Autodesk Inventor part; units mm, degrees
ref_plane "YZ Plane" through (0, 0, 0) normal (1, 0, 0) x (0, 1, 0)
ref_plane "XZ Plane" through (0, 0, 0) normal (0, 1, 0) x (-1, 0, 0)
ref_plane "XY Plane" through (0, 0, 0) normal (0, 0, 1) x (1, 0, 0)
sketch "スケッチ1" plane through (0, 0, 0) normal (0, 0, 1) x (1, 0, 0)
  line L0 (-22.5, -5) -> (22.5, -5)
  line L1 (22.5, -5) -> (22.5, 5)
  line L2 (22.5, 5) -> (-22.5, 5)
  line L3 (-22.5, 5) -> (-22.5, -5)
  line L4 (-22.5, -5) -> (22.5, 5) construction
  line L5 (22.5, -5) -> (-22.5, 5) construction
  point P0 (0, 0)
  dimension "d0" = 45
  dimension "d1" = 10
extrude "押し出し1" add sketch "スケッチ1" along normal mid plane 55
sketch "スケッチ2" plane through (0, 0, 27.5) normal (0, 0, 1) x (1, 0, 0)
  line L0 (22.5, 5) -> (-22.5, 5)
  line L1 (-22.5, 5) -> (-22.5, -5)
  line L2 (22.5, -5) -> (22.5, 5)
  point P0 (0, 0)
  point P1 (-17.5, 0)
  point P2 (17.5, 0)
  dimension "d4" = 5
  dimension "d5" = 5
  dimension "d6" = 5
  dimension "d7" = 5
hole "穴1" at (-17.5, 0, 27.5) at (17.5, 0, 27.5) direction (0, 0, -1) diameter 2.459 depth 8.8 tip angle 118
sketch "スケッチ3" plane through (0, 0, -27.5) normal (0, 0, -1) x (-1, 0, 0)
  line L0 (-22.5, 5) -> (-22.5, -5)
  line L1 (-22.5, -5) -> (22.5, -5)
  line L2 (22.5, -5) -> (22.5, 5)
  line L3 (22.5, 5) -> (-22.5, 5)
  circle A0 centre (-17.5, 0) radius 1.2295
  circle A1 centre (17.5, 0) radius 1.2295
  point P0 (0, 0)
hole "穴2" at (17.5, 0, -27.5) at (-17.5, 0, -27.5) direction (0, 0, 1) diameter 2.459 depth 8.8 tip angle 118
sketch "スケッチ4" plane through (-22.5, 5, 27.5) normal (0, 1, 0) x (1, 0, 0)
  line L0 (45, 55) -> (45, 0)
  line L1 (45, 0) -> (0, 0)
  point P0 (22.5, 27.5)
  point P1 (33, 27.5)
  dimension "d22" = 12
  dimension "d23" = 27.5
hole "穴3" at (10.5, 5, 0) direction (0, -1, 0) diameter 6.4 end through all
sketch "スケッチ5" plane through (0, 0, 27.5) normal (0, 0, 1) x (1, 0, 0)
  circle A0 centre (17.5, 0) radius 1.2295
  circle A1 centre (-17.5, 0) radius 1.2295
  line L0 (22.5, -5) -> (22.5, 5)
  line L1 (22.5, 5) -> (-22.5, 5)
  line L2 (-22.5, 5) -> (-22.5, -5)
  line L3 (-22.5, -5) -> (22.5, -5)
  line L4 (-17.5, 0) -> (17.5, 0) construction
  line L5 (-17.5, -5) -> (17.5, -5)
  line L6 (17.5, 5) -> (-17.5, 5)
  arc A2 (-17.5, 5) -> (-17.5, -5) centre (-17.5, 0) ccw
  arc A3 (17.5, -5) -> (17.5, 5) centre (17.5, 0) ccw
  point P0 (0, 0)
  point P1 (0, 0)
  point P2 (22.5, 0)
  point P3 (-22.5, 0)
extrude "押し出し2" cut sketch "スケッチ5" against normal through all contours L3 A3 L0 | A3 L1 L0 | L3 L2 A2 | A2 L2 L1
properties part number "camera_connect_part"
For this review, take the finished solid that the model builds, in its own axes (mm). A direction names the side the tool comes from. Coordinates: 2 decimals unless noted, no trailing zeros. Loops run counter-clockwise (first coordinate to the right, second up) from the corner with the lowest first, then second, coordinate; pieces in that order, holes last. Notation, with made-up numbers: (77, -0.5) - (99, -0.5) arc R28 cw to (99, 18.5) - close; hole circle Ø10 at (41.25, -23). An arc over 180 degrees is marked (long way). Use a Markdown table: item, result. Add a question column.
Item 1: Tool access review of faces 1 (the face through (7.327, -0.07, -0.417)), 2 (the face through (16.28, -0.16, -23.04)), 3 (the face through (16.28, 0.16, 23.04)): name each direction out of +Z, -Z, +X, -X, +Y, -Y from which nothing blocks a thin tool from reaching the whole face with its end or side.
Item 2: Mouldability with a two-part tool opening along X and no side actions: class faces 4 (the face through (22.5, -0.1, 0.4)), 5 (the face through (0, 5, 0)), 6 (the face through (17.71, -0.03, -18.09)) as pulls with the +X half, pulls with the -X half, needs draft (parallel to the pull), parting line crosses it, or undercut.
Item 3: For line 1 (X direction, y = 0, z = 25.75); line 2 (Y direction, x = -17.5, z = 24.5); line 3 (Z direction, x = 11, y = -1.5), list the stretches that pass through material, from the lowest coordinate up.
Item 4: We need section B-B (z = 0). Give the boundary of the cut face in (x, y).
Item 5: We need section C-C (z = 22.5). Give the boundary of the cut face in (x, y), and give its area (3 significant figures).
Item 6: We need section D-D (y = 2.5). Give the boundary of the cut face in (x, z).
Item 7: We need section A-A (x = 10.5). Give the boundary of the cut face in (y, z).
Results list:
| question | item | result |
|---|---|---|
| 1 | face 1 | +Y, -Y |
| 1 | face 2 | -Z |
| 1 | face 3 | +Z |
| 2 | face 4 | pulls with the +X half |
| 2 | face 5 | needs draft |
| 2 | face 6 | undercut |
| 3 | line 1 | x = -22.5 to -18.73, -16.27 to 16.27, 18.73 to 22.5 |
| 3 | line 2 | y = -5 to -1.23, 1.23 to 5 |
| 3 | line 3 | z = -27.5 to -3.16, 3.16 to 27.5 |
| 4 | outline | (-17.5, -5) - (7.3, -5) - (7.3, 5) - (-17.5, 5) arc R5 ccw to start; (13.7, -5) - (17.5, -5) arc R5 ccw to (17.5, 5) - (13.7, 5) - close |
| 5 | outline | (-17.5, -5) - (17.5, -5) arc R5 ccw to (17.5, 5) - (-17.5, 5) arc R5 ccw to start; hole circle Ø2.46 at (-17.5, 0); hole circle Ø2.46 at (17.5, 0) |
| 5 | area | 419 mm^2 |
| 6 | outline | (-21.83, -27.5) - (21.83, -27.5) - (21.83, 27.5) - (-21.83, 27.5) - close; hole circle Ø6.4 at (10.5, 0) |
| 7 | outline | (-5, -27.5) - (5, -27.5) - (5, -3.2) - (-5, -3.2) - close; (-5, 3.2) - (5, 3.2) - (5, 27.5) - (-5, 27.5) - close |
